Verification items for the finished model (mm, model axes). A direction names the side the tool comes from. Round coordinates to 2 decimals unless told otherwise and drop trailing zeros. Order: outer loops, then holes, each group sorted by start corner. A loop starts at its lowest first (then second) coordinate and runs counter-clockwise, first axis right, second up. Notation, with made-up numbers: M 77.25,29.25 L 104.25,29.25 A34 ccw 104.25,64.25 Z; hole C 32,22.5 d10. An arc over 180 degrees is marked long. Return JSON: item names as keys, results as strings. Group by question number.
from build123d import *

# Parameters (mm, degrees)
SKETCH_W     = 100
SKETCH_H     = 70
PAD_DEPTH    = 50
CHAMFER_SIZE = 31
THICKNESS_T  = -2
SKETCH001_W  = 10
SKETCH001_H  = 66
PAD001_DEPTH = 10
SKETCH002_W  = 22.304644
SKETCH002_H  = 12.181445
POCKET_DEPTH = 11
FILLET_R     = 1


with BuildPart() as part:
    # Sketch → Pad (new body)
    with BuildSketch(Plane.XY):
        Rectangle(SKETCH_W, SKETCH_H)
    extrude(amount=PAD_DEPTH)

    # Chamfer
    chamfer_edges = [part.edges().sort_by_distance(p)[0] for p in [
        (0, -35, 50),
    ]]
    chamfer(chamfer_edges, length=CHAMFER_SIZE)

    # Thickness
    thickness_openings = [part.faces().sort_by_distance(p)[0] for p in [
        (0, 15.5, 50),
        (0, -19.5, 34.5),
    ]]
    offset(amount=THICKNESS_T, openings=thickness_openings)

    # Sketch001 (on Face12 of Thickness) → Pad001 (join)
    with BuildSketch(Plane.XY.offset(2)):
        Rectangle(SKETCH001_W, SKETCH001_H)
    extrude(amount=PAD001_DEPTH)

    # Sketch002 (on Face1 of Pad001) → Pocket (cut)
    with BuildSketch(Plane.XZ.offset(35)):
        with Locations((22.553599, 14.909277)):
            Rectangle(SKETCH002_W, SKETCH002_H)
    extrude(amount=-POCKET_DEPTH, mode=Mode.SUBTRACT)

    # Fillet
    fillet_edges = [part.edges().sort_by_distance(p)[0] for p in [
        (33.705921, -34, 8.818555),
        (11.401277, -34, 8.818555),
    ]]
    fillet(fillet_edges, radius=FILLET_R)


solid = part.part
1. Cross-section at A-A (z = 25.5). Enter the section's corners in (x, y).
2. Cross-section at D-D (x = 1). Enter the section's corners in (y, z).
3. Access from +Z, -Z, +X, -X, +Y, -Y to the whole of each face (thin tool, end or side, straight path). Record for faces 1 (the face through (-1, 33, 26)), 2 (the face through (11.401, -34, 15)), 3 (the face through (-1, 0, 0)).
4. Thickness scan on line 1 along X through (y, z) = (13, 9); line 2 along Y through (x, z) = (37, 10); line 3 along X through (y, z) = (24.5, 19). Record the ranges inside material, lowest first. Write a range as from..to.
5. Cross-section at C-C (z = 7.5). Enter the section's corners in (x, y), plus the area to 3 significant figures.
6. Go/stop test with flat-tipped pins: pin 1 (3 mm diameter, centred on x = 28.5, y = 27.5, fed in from -Z); pin 2 (13 mm diameter, centred on x = -34.5, y = -5.5, fed in from +Z); pin 3 (2 mm diameter, centred on x = 20, y = -33.5, fed in from +Z); pin 4 (3 mm diameter, centred on x = 6, y = -24, fed in from +Z). Record where each tip stops, or that it passes through.
7. Cross-section at B-B (y = -12). Enter the section's corners in (x, z).
Computed:
{
 "1": {"outline": "M -50,-28.5 L -48,-28.5 L -48,33 L 48,33 L 48,-28.5 L 50,-28.5 L 50,35 L -50,35 Z"},
 "2": {"outline": "M -35,0 L 35,0 L 35,50 L 33,50 L 33,12 L -33,12 L -33,21 L -35,19 Z"},
 "3": {"face 1": "+Z", "face 2": "+Z, -Y", "face 3": "-Z, +X, -X, +Y, -Y"},
 "4": {"line 1": "x = -50..-48, -5..5, 48..50", "line 2": "y = -35..-33, 33..35", "line 3": "x = -50..-48, 48..50"},
 "5": {"outline": "M -50,-35 L 50,-35 L 50,35 L -50,35 Z; hole M -48,-33 L -5,-33 L -5,33 L -48,33 Z; hole M 5,-33 L 48,-33 L 48,33 L 5,33 Z", "area": "1,320 mm²"},
 "6": {"pin 1": "stops at z = 0", "pin 2": "stops at z = 2", "pin 3": "stops at z = 8.82", "pin 4": "stops at z = 12"},
 "7": {"outline": "M -50,0 L 50,0 L 50,42 L 48,42 L 48,2 L 5,2 L 5,12 L -5,12 L -5,2 L -48,2 L -48,42 L -50,42 Z"}
}
